The listing builds one solid part. Answer for the finished solid, in the listing's coordinates (mm). Give positions to 0.01 mm unless a question says otherwise; leave off trailing zeros. Loops run counter-clockwise (first coordinate to the right, second up) from the corner with the lowest first, then second, coordinate; pieces in that order, holes last. Notation, with made-up numbers: (47.5, 50) - (65.5, 50) arc R20 ccw to (65.5, 72) - close; hole circle Ø2 at (34.5, 59). An arc over 180 degrees is marked (long way). Answer as CSV lines item,"result". Start each with the question number.
1) A cutting plane is placed at B-B (y = -23.5). Determine the outline of the cut face in (x, z).
2) A cutting plane is placed at C-C (x = -8.25). Determine the outline of the cut face in (y, z).
3) A cutting plane is placed at A-A (x = -20). Determine the outline of the cut face in (y, z), and give its area (3 significant figures).
4) Find the intervals of material crossed by line 1 along Y through (x, z) = (-8.25, 0.4); line 2 along Y through (x, z) = (-21.5, 0.4); line 3 along X through (y, z) = (-25, 0.3), in increasing order.
5) A cutting plane is placed at D-D (z = 0.4). Give the number of separate pieces and of enclosed holes in the cut face, and give its area (3 significant figures).
6) Flat-ended cylindrical pins translate along their axes: pin 1 (1 mm diameter, centred on x = -10.75, y = 9.79, fed in from -Z); pin 2 (0.5 mm diameter, centred on x = -16.5, z = 0.5, fed in from -Y); pin 3 (1.9 mm diameter, centred on x = 1.35, y = -18.79, fed in from -Z). Find the tip coordinate at first contact, or state that the pin passes through.
```python
from build123d import *

# Parameters (mm, degrees)
BOARD_DEPTH        = 1
ESC_DEPTH          = 60.97841413
HOLE1SKE_R         = 0.5
HOLE1SKE_R_2       = 2.5
HOLE1_DEPTH        = 60.97841413
HOLE2SKE_R         = 1
HOLE2_DEPTH        = 60.97841413
HOLE3SKE_R         = 0.5
HOLE3_DEPTH        = 60.97841413
MOTORSETSKE_R      = 2
MOTORSET_DEPTH     = 60.97841413
MOTORSETHOLESKE_R  = 0.6
MOTORSETHOLE_DEPTH = 60.97841413


with BuildPart() as part:
    # BoardSke → Board (new body)
    with BuildSketch(Plane.XY):
        with BuildLine():
            Line((42.5, 4.330127019), (-17.5, 38.97114317))
            ThreePointArc((-17.5, 38.97114317), (-22.5, 38.97114317), (-25, 34.641016151))
            Line((-25, 34.641016151), (-25, -34.641016151))
            ThreePointArc((-25, -34.641016151), (-22.5, -38.97114317), (-17.5, -38.97114317))
            Line((-17.5, -38.97114317), (42.5, -4.330127019))
            ThreePointArc((42.5, -4.330127019), (45, 0), (42.5, 4.330127019))
        make_face()
    extrude(amount=BOARD_DEPTH)

    # ESCSke → ESC (cut, through all)
    with BuildSketch(Plane.XY.offset(1)):
        Polygon((-6.65, -30), (-21.9, -30), (-21.9, -21.951), (-5.95, -21.951), (-5.95, -29.6), align=None)
    extrude(amount=-ESC_DEPTH, mode=Mode.SUBTRACT)

    # Hole1Ske → Hole1 (cut, through all)
    with BuildSketch(Plane.XY.offset(1)):
        with Locations((-6, 0)):
            Circle(HOLE1SKE_R)
        with Locations((3, 5.196152423)):
            Circle(HOLE1SKE_R)
        with Locations((3, -5.196152423)):
            Circle(HOLE1SKE_R)
        Circle(HOLE1SKE_R_2)
    extrude(amount=-HOLE1_DEPTH, mode=Mode.SUBTRACT)

    # Hole2Ske → Hole2 (cut, through all)
    with BuildSketch(Plane.XY.offset(1)):
        with Locations((40, 0)):
            Circle(HOLE2SKE_R)
        with Locations((-20, -34.641016151)):
            Circle(HOLE2SKE_R)
        with Locations((-20, 34.641016151)):
            Circle(HOLE2SKE_R)
    extrude(amount=-HOLE2_DEPTH, mode=Mode.SUBTRACT)

    # Hole3Ske → Hole3 (cut, through all)
    with BuildSketch(Plane.XY.offset(1)):
        with Locations((40, 3)):
            Circle(HOLE3SKE_R)
        with Locations((40, -3)):
            Circle(HOLE3SKE_R)
        with Locations((-22.598076211, -33.141016151)):
            Circle(HOLE3SKE_R)
        with Locations((-17.401923789, -36.141016151)):
            Circle(HOLE3SKE_R)
        with Locations((-17.401923789, 36.141016151)):
            Circle(HOLE3SKE_R)
        with Locations((-22.598076211, 33.141016151)):
            Circle(HOLE3SKE_R)
        with Locations((43, 0)):
            Circle(HOLE3SKE_R)
        with Locations((-21.5, -37.239092363)):
            Circle(HOLE3SKE_R)
        with Locations((-21.5, 37.239092363)):
            Circle(HOLE3SKE_R)
    extrude(amount=-HOLE3_DEPTH, mode=Mode.SUBTRACT)

    # MotorSetSke → MotorSet (cut, through all)
    with BuildSketch(Plane.XY.offset(1)):
        with Locations((-8.25, 14.289419162)):
            Circle(MOTORSETSKE_R)
    motorset = extrude(amount=-MOTORSET_DEPTH, mode=Mode.SUBTRACT)

    # MotorSetHoleSke → MotorSetHole (cut, through all)
    with BuildSketch(Plane.XY.offset(1)):
        with Locations((-10.754495957, 18.789419162)):
            Circle(MOTORSETHOLESKE_R)
        with Locations((-10.754495957, 9.789419162)):
            Circle(MOTORSETHOLESKE_R)
        with Locations((1.345504043, 18.789419162)):
            Circle(MOTORSETHOLESKE_R)
    motorsethole = extrude(amount=-MOTORSETHOLE_DEPTH, mode=Mode.SUBTRACT)

    # Mirror 2: MotorSet, MotorSetHole across plane
    add(motorset.mirror(Plane.ZX), mode=Mode.SUBTRACT)
    add(motorsethole.mirror(Plane.ZX), mode=Mode.SUBTRACT)


solid = part.part
```
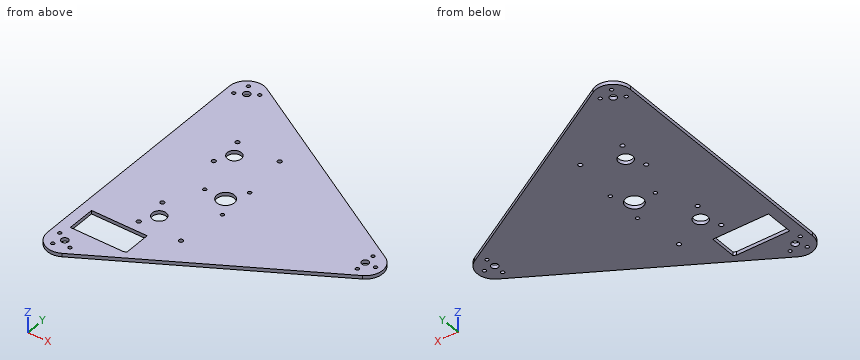
Ans:
1,outline,"(-25, 0) - (-21.9, 0) - (-21.9, 1) - (-25, 1) - close; (-5.95, 0) - (9.3, 0) - (9.3, 1) - (-5.95, 1) - close"
2,outline,"(-33.63, 0) - (-30, 0) - (-30, 1) - (-33.63, 1) - close; (-21.95, 0) - (-16.29, 0) - (-16.29, 1) - (-21.95, 1) - close; (-12.29, 0) - (12.29, 0) - (12.29, 1) - (-12.29, 1) - close; (16.29, 0) - (33.63, 0) - (33.63, 1) - (16.29, 1) - close"
3,outline,"(-39.64, 0) - (-35.64, 0) - (-35.64, 1) - (-39.64, 1) - close; (-33.64, 0) - (-30, 0) - (-30, 1) - (-33.64, 1) - close; (-21.95, 0) - (33.64, 0) - (33.64, 1) - (-21.95, 1) - close; (35.64, 0) - (39.64, 0) - (39.64, 1) - (35.64, 1) - close"
3,area,"67.2 mm2"
4,line 1,"-33.63 to -30, -21.95 to -16.29, -12.29 to 12.29, 16.29 to 33.63"
4,line 2,"-39.41 to -37.74, -36.74 to -30, -21.95 to 36.74, 37.74 to 39.41"
4,line 3,"-25 to -21.9, -5.95 to 6.7"
5,separate pieces,"1"
5,enclosed holes,"25"
5,area,"3,000 mm2"
6,pin 1,"through"
6,pin 2,"y = -38.54"
6,pin 3,"z = 0"
